Geometry check sheet. Reference: the model listing, model coordinates, mm. A direction names the side the tool comes from. Give positions to 0.01 mm unless a question says otherwise; leave off trailing zeros. Loops run counter-clockwise (first coordinate to the right, second up) from the corner with the lowest first, then second, coordinate; pieces in that order, holes last.
1. Cross-section at C-C, the plane x = 37. Record the cut outline in (y, z) (3 decimals).
2. Material ranges on L1, parallel to X at y = 47, z = -2; L2, parallel to X at y = 12, z = -29; L3, parallel to Y at x = -5, z = -1.55, recorded low to high.
3. Go/stop test with flat-tipped pins: pin 1 Ø7.5 at (x, y) = (37.5, 3.5) entering from +Z; pin 2 Ø1 at (y, z) = (10, -29.5) entering from -X; pin 3 Ø11 at (x, y) = (-5, 7.5) entering from -Z (3 decimals); pin 4 Ø10 at (y, z) = (20, -20.5) entering from -X. Record where each tip stops, or that it passes through.
4. Cross-section at B-B, the plane y = 12.42. Record the cut outline in (x, z) (3 decimals), plus the area to 3 significant figures.
5. Cross-section at A-A, the plane y = 47.42. Record the cut outline in (x, z) (3 decimals).
6. Release check for a two-part mould opening along X. For faces 4 (the flat face through (-5, 52.5, -2)), 5 (the cylindrical face through (-9.49, -4.65, -1.61)), 6 (the cylindrical face through (34.654, 11.447, -30.26)) record: +X half, -X half, draft (parallel to the pull), parting line (faces both ways), or undercut.
7. Cross-section at D-D, the plane z = -30. Record the cut outline in (x, y).
8. Tool access check on faces 1 (the flat face through (12.5, 0, -16)), 2 (the flat face through (15, 7.5, -17)), 3 (the flat face through (31, 2, -31.825)). Record the directions out of +Z, -Z, +X, -X, +Y, -Y that give a thin tool (end or side, any length) a straight path to the whole face; none if there is none.
from build123d import *

# Parameters (mm, degrees)
SKETCH1_W                    = 25
SKETCH1_H                    = 15
BASE_FLANGE1_DEPTH           = 3.175
EDGE_FLANGE1_STRIP_W         = 18.7
EDGE_FLANGE1_STRIP_H         = 3.175
EDGE_FLANGE1_STRIP_CUT_DEPTH = 15
EDGE_FLANGE1_DEPTH           = 15
EDGE_FLANGE2_STRIP_W         = 18.7
EDGE_FLANGE2_STRIP_H         = 3.175
EDGE_FLANGE2_STRIP_CUT_DEPTH = 15
EDGE_FLANGE2_DEPTH           = 15
SKETCH12_W                   = 15
SKETCH12_H                   = 3.175
BOSS_EXTRUDE1_DEPTH          = 45
SKETCH15_R                   = 2.54
CUT_EXTRUDE2_DEPTH           = 75.547451331
SKETCH19_W                   = 15
SKETCH19_H                   = 3.175
BOSS_EXTRUDE2_DEPTH          = 10
SKETCH21_R                   = 2.54
CUT_EXTRUDE3_DEPTH           = 76.824340584
FILLET2_R                    = 3
FILLET3_R                    = 10


# Sheet-metal steps are written as plain solids
with BuildPart() as part:
    # Sketch1 → Base-Flange1 (new body)
    with BuildSketch(Plane.XY):
        Rectangle(SKETCH1_W, SKETCH1_H)
    extrude(amount=-BASE_FLANGE1_DEPTH)

    # Edge-Flange1 strip (across the edge) → Edge-Flange1 strip cut (cut)
    with BuildSketch(Plane(origin=(12.5, 7.5, -3.175), x_dir=(-1, 0, 0), z_dir=(0, -1, 0))):
        with Locations((-6.35, -1.5875)):
            Rectangle(EDGE_FLANGE1_STRIP_W, EDGE_FLANGE1_STRIP_H)
    extrude(amount=EDGE_FLANGE1_STRIP_CUT_DEPTH, mode=Mode.SUBTRACT)

    # Edge-Flange1 section (across the edge) → Edge-Flange1 (add)
    with BuildSketch(Plane(origin=(12.5, 7.5, -3.175), x_dir=(-1, 0, 0), z_dir=(0, -1, 0))):
        with BuildLine():
            Line((-3.175, 3), (-3.175, 25.475))
            Line((-3.175, 25.475), (0, 25.475))
            Line((0, 25.475), (0, 3))
            ThreePointArc((0, 3), (0.878679656, 0.878679656), (3, 0))
            Line((3, 0), (3, -3.175))
            ThreePointArc((3, -3.175), (-1.366384374, -1.366384374), (-3.175, 3))
        make_face()
    extrude(amount=EDGE_FLANGE1_DEPTH)

    # Edge-Flange2 strip (across the edge) → Edge-Flange2 strip cut (cut)
    with BuildSketch(Plane(origin=(15.675, -7.5, -28.65), x_dir=(0, 0, 1), z_dir=(0, 1, 0))):
        with Locations((-6.35, -1.5875)):
            Rectangle(EDGE_FLANGE2_STRIP_W, EDGE_FLANGE2_STRIP_H)
    extrude(amount=EDGE_FLANGE2_STRIP_CUT_DEPTH, mode=Mode.SUBTRACT)

    # Edge-Flange2 section (across the edge) → Edge-Flange2 (add)
    with BuildSketch(Plane(origin=(15.675, -7.5, -28.65), x_dir=(0, 0, 1), z_dir=(0, 1, 0))):
        with BuildLine():
            Line((-3.175, 3), (-3.175, 28.825))
            Line((-3.175, 28.825), (0, 28.825))
            Line((0, 28.825), (0, 3))
            ThreePointArc((0, 3), (0.878679656, 0.878679656), (3, 0))
            Line((3, 0), (3, -3.175))
            ThreePointArc((3, -3.175), (-1.366384374, -1.366384374), (-3.175, 3))
        make_face()
    extrude(amount=EDGE_FLANGE2_DEPTH)

    # Sketch12 → Boss-Extrude1 (add)
    with BuildSketch(Plane(origin=(0, 7.5, 0), x_dir=(1, 0, 0), z_dir=(0, 1, 0))):
        with Locations((-5, 1.5875)):
            Rectangle(SKETCH12_W, SKETCH12_H)
    extrude(amount=BOSS_EXTRUDE1_DEPTH)

    # Sketch15 → Cut-Extrude2 (cut, through all)
    with BuildSketch(Plane(origin=(0, 0, -3.175), x_dir=(-1, 0, 0), z_dir=(0, 0, -1))):
        with Locations((5, 47.42)):
            Circle(SKETCH15_R)
    extrude(amount=-CUT_EXTRUDE2_DEPTH, mode=Mode.SUBTRACT)

    # Sketch19 → Boss-Extrude2 (add)
    with BuildSketch(Plane(origin=(0, 7.5, 0), x_dir=(1, 0, 0), z_dir=(0, 1, 0))):
        with Locations((37, 30.2375)):
            Rectangle(SKETCH19_W, SKETCH19_H)
    extrude(amount=BOSS_EXTRUDE2_DEPTH)

    # Sketch21 → Cut-Extrude3 (cut, through all)
    with BuildSketch(Plane(origin=(0, 0, -31.825), x_dir=(-1, 0, 0), z_dir=(0, 0, -1))):
        with Locations((-37, 12.42)):
            Circle(SKETCH21_R)
    extrude(amount=-CUT_EXTRUDE3_DEPTH, mode=Mode.SUBTRACT)

    # Fillet2
    fillet2_edges = [part.edges().sort_by_distance(p)[0] for p in [
        (44.5, 17.5, -30.2375),
        (29.5, 17.5, -30.2375),
        (-12.5, 52.5, -1.5875),
        (2.5, 52.5, -1.5875),
    ]]
    fillet(fillet2_edges, radius=FILLET2_R)

    # Fillet3
    fillet3_edges = [part.edges().sort_by_distance(p)[0] for p in [
        (44.5, -7.5, -30.2375),
        (-12.5, -7.5, -1.5875),
    ]]
    fillet(fillet3_edges, radius=FILLET3_R)


solid = part.part
Result:
1. outline: (-7.182, -31.825) - (9.88, -31.825) - (9.88, -28.65) - (-7.182, -28.65) - close; (14.96, -31.825) - (17.5, -31.825) - (17.5, -28.65) - (14.96, -28.65) - close
2. L1: x = -12.5 to -7.51, -2.49 to 2.5
2. L2: x = 29.5 to 34.49, 39.51 to 44.5
2. L3: y = -7.18 to 44.88, 49.96 to 52.5
3. pin 1: stops at z = -28.65
3. pin 2: stops at x = 29.5
3. pin 3: stops at z = -3.175
3. pin 4: passes through
4. outline: (-12.5, -3.175) - (2.5, -3.175) - (2.5, 0) - (-12.5, 0) - close; (29.5, -31.825) - (34.46, -31.825) - (34.46, -28.65) - (29.5, -28.65) - close; (39.54, -31.825) - (44.5, -31.825) - (44.5, -28.65) - (39.54, -28.65) - close
4. area: 79.1 mm2
5. outline: (-12.5, -3.175) - (-7.54, -3.175) - (-7.54, 0) - (-12.5, 0) - close; (-2.46, -3.175) - (2.5, -3.175) - (2.5, 0) - (-2.46, 0) - close
6. face 4: draft
6. face 5: -X half
6. face 6: undercut
7. outline: (14.29, -7.5) - (34.5, -7.5) arc R10 ccw to (44.5, 2.5) - (44.5, 14.5) arc R3 ccw to (41.5, 17.5) - (32.5, 17.5) arc R3 ccw to (29.5, 14.5) - (29.5, 7.5) - (14.29, 7.5) - close; hole circle Ø5.08 at (37, 12.42)
8. face 1: -Z, -X, +Y, -Y
8. face 2: +Z, -Z, +Y
8. face 3: -Z, +X, -X, +Y, -Y
